```python
from build123d import *

# Parameters (mm, degrees)
EXTRUDE_1_DEPTH = 117
EXTRUDE_2_DEPTH = 1.5
EXTRUDE_3_DEPTH = 1.5
EXTRUDE_START   = -6
EXTRUDE_4_DEPTH = 108
EXTRUDE_5_DEPTH = 108
FILLET_1_R      = 0.1
FILLET_2_R      = 0.2


with BuildPart() as part:
    # 草图1 → 凸台-拉伸1 (new body)
    with BuildSketch(Plane(origin=(0, 0, 0), x_dir=(0, 0, -1), z_dir=(1, 0, 0))):
        Polygon((0, 0), (-40, 0), (-45.5, 0), (-41, 1.5), (-40, 1.5), (-1.5, 1.5), (-1.5, 14.598076211), (-17.299038106, 41.962812921), (-16, 42.712812921), (0, 15), align=None)
    extrude(amount=EXTRUDE_1_DEPTH)

    # 草图2 → 凸台-拉伸2 (add)
    with BuildSketch(Plane(origin=(117, 0, 0), x_dir=(0, 0, -1), z_dir=(1, 0, 0))):
        Polygon((-41, 1.5), (-40, 1.5), (-17.299038106, 41.962812921), (-16, 42.712812921), (0, 15), (0, 0), (-45.5, 0), align=None)
    extrude(amount=EXTRUDE_2_DEPTH)

    # 草图3 → 凸台-拉伸3 (add)
    with BuildSketch(Plane.ZY):
        Polygon((41, 1.5), (40, 1.5), (17.299038106, 41.962812921), (16, 42.712812921), (0, 15), (0, 0), (45.5, 0), align=None)
    extrude(amount=EXTRUDE_3_DEPTH)

    # 草图4 → 凸台-拉伸4 (add)
    with BuildSketch(Plane.ZY.offset(1.5).offset(EXTRUDE_START)):
        with BuildLine():
            Line((0, 7.5), (0, 6))
            Line((0, 6), (-0.677124344, 6))
            ThreePointArc((-0.677124344, 6), (-1.088161527, 5.719957697), (-1.555590279, 5.55))
            Line((-1.555590279, 5.55), (-2.5, 5.55))
            Line((-2.5, 5.55), (-2.5, 6.056624327))
            Line((-2.5, 6.056624327), (0, 7.5))
        make_face()
    extrude_4 = extrude(amount=-EXTRUDE_4_DEPTH)

    # 镜向1: 凸台-拉伸4 across plane
    add(extrude_4.mirror(Plane(origin=(0, 7.5, 0), x_dir=(0, 0, 1), z_dir=(0, -1, 0))))

    # 草图5 → 凸台-拉伸5 (add)
    with BuildSketch(Plane.ZY.offset(1.5).offset(EXTRUDE_START)):
        with BuildLine():
            Line((3.75, 21.495190528), (4.5, 22.794228634))
            Line((4.5, 22.794228634), (3.913593116, 23.132790806))
            ThreePointArc((3.913593116, 23.132790806), (3.697645625, 23.580833146), (3.3778193, 23.961735205))
            Line((3.3778193, 23.961735205), (2.559936491, 24.433940066))
            Line((2.559936491, 24.433940066), (2.306624327, 23.995190528))
            Line((2.306624327, 23.995190528), (3.75, 21.495190528))
        make_face()
    extrude_5 = extrude(amount=-EXTRUDE_5_DEPTH)

    # 镜向2: 凸台-拉伸5 across plane
    add(extrude_5.mirror(Plane(origin=(0, 17.745190528, 10.245190528), x_dir=(0, -0.49999999999999695, 0.8660254037844404), z_dir=(0, 0.8660254037844406, 0.49999999999999684))))

    # 圆角1
    fillet_1_edges = [part.edges().sort_by_distance(p)[0] for p in [
        (112.5, 24.214565297, 2.433280409),
        (58.5, 23.995190528, 2.306624327),
        (58.5, 24.433940066, 2.559936491),
        (4.5, 24.214565297, 2.433280409),
        (58.5, 21.495190528, 0.863248654),
        (4.5, 21.27581576, 0.736592572),
        (58.5, 21.056440991, 0.609936491),
        (112.5, 21.27581576, 0.736592572),
        (58.5, 6.056624327, -2.5),
        (112.5, 5.803312164, -2.5),
        (58.5, 5.55, -2.5),
        (4.5, 5.803312164, -2.5),
        (4.5, 9.196687836, -2.5),
        (58.5, 8.943375673, -2.5),
        (58.5, 9.45, -2.5),
        (112.5, 9.196687836, -2.5),
    ]]
    fillet(fillet_1_edges, radius=FILLET_1_R)

    # 圆角2
    fillet_2_edges = [part.edges().sort_by_distance(p)[0] for p in [
        (118.5, 0.75, 43.25),
        (118.5, 1.5, 40.5),
        (118.5, 21.731406461, 28.649519053),
        (118.5, 42.337812921, 16.649519053),
        (118.5, 28.856406461, 8),
        (118.5, 7.5, 0),
        (118.5, 0, 22.75),
        (-1.5, 42.337812921, 16.649519053),
        (-1.5, 21.731406461, 28.649519053),
        (-1.5, 1.5, 40.5),
        (-1.5, 0.75, 43.25),
        (-1.5, 0, 22.75),
        (-1.5, 7.5, 0),
        (-1.5, 28.856406461, 8),
        (58.5, 0, 0),
        (58.5, 15, 0),
        (58.5, 42.712812921, 16),
    ]]
    fillet(fillet_2_edges, radius=FILLET_2_R)


solid = part.part
```
Part model, mm, in its own coordinate system. A direction names the side the tool comes from. Round coordinates to 2 decimals unless told otherwise and drop trailing zeros.
Item 1: Drill centre lines: line 1 (X direction, y = 8, z = 14); line 2 (Y direction, x = 51.5, z = 28); line 3 (Y direction, x = 9, z = 2). Where is each one in solid material? Low to high.
Item 2: 3-axis set-ups, long thin cutter, end or side, ignore diameter. For faces 4 (the face through (59, 1.5, 22)), 5 (the face through (4.5, 23, 3.4)), 6 (the face through (117.641, 21.448, 28.808)): which of +Z, -Z, +X, -X, +Y, -Y reach the whole face in a straight line?
Item 3: Mould opens along Y. For faces 1 (the face through (59, 0, 23)), 2 (the face through (-1.5, 17, 17)), 3 (the face through (57.744, 6.783, -1.242)) say: +Y half, -Y half, draft (parallel to the pull), parting line (faces both ways), or undercut.
Item 4: Drop flat-ended pins along their axis: P1, Ø8, axis at x = 18.5, y = 6, coming from the +Z side; P2, Ø4.5, axis at x = 84, y = 10, coming from the -Z side; P3, Ø1.6, axis at y = 6.5, z = -1.5, coming from the +X side; P4, Ø1.5, axis at x = 35.5, y = 15.5, coming from the -Z side. Give the stop position or say it passes through.
A:
1. line 1: x = -1.5 to 0, 117 to 118.5
1. line 2: y = 0 to 1.5
1. line 3: y = 0 to 1.5, 15.46 to 18.46, 20.5 to 21.5
2. face 4: +Z
2. face 5: -Z, -X, +Y
2. face 6: +Z, +X, -X, +Y
3. face 1: -Y half
3. face 2: draft
3. face 3: undercut
4. P1: stops at z = 1.5
4. P2: stops at z = -2.5
4. P3: stops at x = 112.5
4. P4: stops at z = 0
